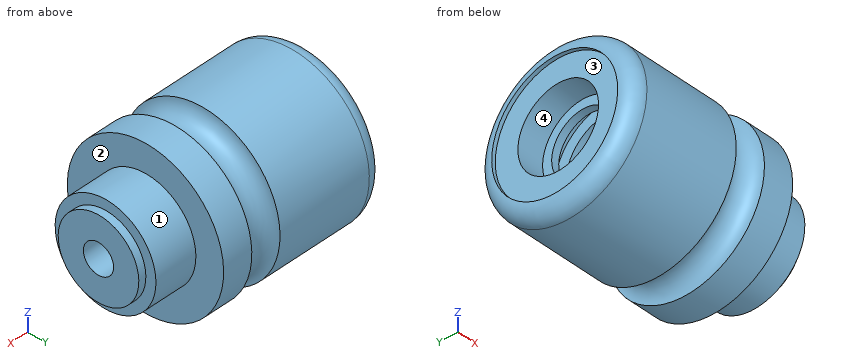
```python
from build123d import *

# Parameters (mm, degrees)
F0_W   = 3
F0_H   = 16
F2_W   = 3
F2_H   = 12.4045886115
F2_W_2 = 58
F2_H_2 = 6


with BuildPart() as f1:
    # F0 (on Front) → F1 (revolve)
    with BuildSketch(Plane.XZ):
        with BuildLine():
            Line((0, 25), (0, 0))
            Line((0, 0), (44, 0))
            Line((44, 0), (44, 31))
            Line((44, 31), (6, 31))
            ThreePointArc((6, 31), (1.7573593129, 29.2426406871), (0, 25))
        make_face()
        with BuildLine():
            Line((44, 31), (44, 0))
            Line((44, 0), (56, 0))
            Line((56, 0), (56, 31))
            ThreePointArc((56, 31), (50, 25), (44, 31))
        make_face()
        Polygon((56, 31), (56, 0), (68, 0), (68, 20), (68, 31), align=None)
        Polygon((68, 20), (68, 0), (85, 0), (85, 16), (85, 20), align=None)
        with Locations((86.5, 8)):
            Rectangle(F0_W, F0_H)
    revolve(axis=Axis((44, 0, 0), (1, 0, 0)))

    # F2 (on Front) → F3 (revolve, cut)
    with BuildSketch(Plane.XZ):
        Polygon((0, 25), (0, 0), (1.5, 0), (1.5, 16), (1.5, 25), align=None)
        Polygon((1.5, 16), (1.5, 0), (12, 0), (12, 12.4045886115), (12, 16), align=None)
        with Locations((13.5, 6.2022943057)):
            Rectangle(F2_W, F2_H)
        Polygon((15, 12.4045886115), (15, 0), (22, 0), (22, 16), (22, 20.5), (15, 20.5), align=None)
        Polygon((22, 16), (22, 0), (30, 0), (30, 6), (30, 16), align=None)
        with Locations((59, 3)):
            Rectangle(F2_W_2, F2_H_2)
    revolve(axis=Axis((44, 0, 0), (1, 0, 0)), mode=Mode.SUBTRACT)


solid = f1.part
```
Design review of the part built by this model. Coordinates are the model's own, in mm. Face numbers are marked on the shaded views. Coordinates: 2 decimals unless noted, no trailing zeros. Loops run counter-clockwise (first coordinate to the right, second up) from the corner with the lowest first, then second, coordinate; pieces in that order, holes last.
Q1. To check wall thickness, follow line 1 (Z direction, x = 27, y = 0); line 2 (Z direction, x = 18, y = 0). State the ranges of each line that lie inside material, in increasing order.
Reported:
line 1: z = -31 to -16, 16 to 31
line 2: z = -31 to -20.5, 20.5 to 31
Q2. We need section A-A on x = 16. State the section outline as (y, z) points, and give its area (3 significant figures).
Reported:
outline: circle Ø62 at (0, 0); hole circle Ø41 at (0, 0)
area: 1,700 mm2
Q3. We need section B-B on x = 80.5. State the section outline as (y, z) points, and give its area (3 significant figures).
Reported:
outline: circle Ø40 at (0, 0); hole circle Ø12 at (0, 0)
area: 1,140 mm2
Q4. The part is to be moulded in two halves that separate along Z. For the marked faces 1, 2, 3 and 4, say which applies: +Z half, -Z half, draft (parallel to the pull), parting line (faces both ways), or undercut.
Reported:
face 1: parting line
face 2: draft
face 3: undercut
face 4: undercut
Q5. For pin 1 (24.5 mm diameter, centred on y = 0, z = 0, fed in from -X); pin 2 (2 mm diameter, centred on x = 46, y = -5, fed in from -Z); pin 3 (16 mm diameter, centred on y = 5.5, z = -8, fed in from -X), all flat-tipped, find the tip position at first contact; note any pin that passes through.
Reported:
pin 1: stops at x = 30
pin 2: stops at z = -27.24
pin 3: stops at x = 1.5
